Check sheet for the modelled part. Datum: model origin and axes. Units: mm. A direction names the side the tool comes from. Coordinates: 2 decimals unless noted, no trailing zeros. Loops run counter-clockwise (first coordinate to the right, second up) from the corner with the lowest first, then second, coordinate; pieces in that order, holes last. Notation, with made-up numbers: M -25,53 L -10,53 A26 ccw -10,92 Z; hole C -29,20 d11. An arc over 180 degrees is marked long. Write each question's results on one line, items separated by ' | '. Start each with the question number.
from build123d import *

# Parameters (mm, degrees)
BOSS_EXTRUDE1_DEPTH = 415.925
SKETCH2_R           = 3.429
CUT_EXTRUDE1_DEPTH  = 26.4


with BuildPart() as part:
    # Sketch1 → Boss-Extrude1 (new body)
    with BuildSketch(Plane.XY):
        with BuildLine():
            Line((-12.446, -12.7), (12.446, -12.7))
            ThreePointArc((12.446, -12.7), (12.625605122, -12.625605122), (12.7, -12.446))
            Line((12.7, -12.446), (12.7, 12.446))
            ThreePointArc((12.7, 12.446), (12.625605122, 12.625605122), (12.446, 12.7))
            Line((12.446, 12.7), (-12.446, 12.7))
            ThreePointArc((-12.446, 12.7), (-12.625605122, 12.625605122), (-12.7, 12.446))
            Line((-12.7, 12.446), (-12.7, -12.446))
            ThreePointArc((-12.7, -12.446), (-12.625605122, -12.625605122), (-12.446, -12.7))
        make_face()
        with BuildLine():
            Line((-11.1125, -9.5885), (-11.1125, 9.5885))
            ThreePointArc((-11.1125, 9.5885), (-10.666130735, 10.666130735), (-9.5885, 11.1125))
            Line((-9.5885, 11.1125), (9.5885, 11.1125))
            ThreePointArc((9.5885, 11.1125), (10.666130735, 10.666130735), (11.1125, 9.5885))
            Line((11.1125, 9.5885), (11.1125, -9.5885))
            ThreePointArc((11.1125, -9.5885), (10.666130735, -10.666130735), (9.5885, -11.1125))
            Line((9.5885, -11.1125), (-9.5885, -11.1125))
            ThreePointArc((-9.5885, -11.1125), (-10.666130735, -10.666130735), (-11.1125, -9.5885))
        make_face(mode=Mode.SUBTRACT)
    extrude(amount=BOSS_EXTRUDE1_DEPTH)

    # Sketch2 → Cut-Extrude1 (cut, through all)
    with BuildSketch(Plane.ZY.offset(12.7)):
        with Locations((371.475, 0)):
            Circle(SKETCH2_R)
        with Locations((358.775, 0)):
            Circle(SKETCH2_R)
        with Locations((346.075, 0)):
            Circle(SKETCH2_R)
        with Locations((12.7, 0)):
            Circle(SKETCH2_R)
        with Locations((25.4, 0)):
            Circle(SKETCH2_R)
        Polygon((415.925, 12.7), (371.930909488, -12.7), (415.925, -12.7), align=None)
        Polygon((0, 5.78069553), (4.844949149, 12.7), (0, 12.7), align=None)
    extrude(amount=-CUT_EXTRUDE1_DEPTH, mode=Mode.SUBTRACT)


solid = part.part
Item 1: Section check D-D (y = 0). State how many separate pieces and enclosed holes the cut face has, plus the area to 3 significant figures.
Item 2: Depth check by flat-ended pin: P1, Ø9, axis at y = 0, z = 346.075, coming from the -X side. Enter the tip coordinate at first touch or a pass-through.
Item 3: Section check B-B (x = -0.75). Record the cut outline in (y, z) (1 decimal).
Item 4: Thickness scan on line 1 (Y direction, x = 8, z = 144); line 2 (Y direction, x = 8, z = 375). Record the ranges inside material, lowest first.
Item 5: Release check for a two-part mould opening along Y. For faces 3 (the face through (-12.7, 0, 205)), 4 (the face through (0, 12.7, 208)), 5 (the face through (11.112, 0, 202)), 6 (the face through (-11.35, 0.06, 394.03)) record: +Y half, -Y half, draft (parallel to the pull), parting line (faces both ways), or undercut.
Item 6: Tool access check on faces 1 (the face through (-11.112, 0, 202)), 2 (the face through (-11.917, -1.313, 361.943)). Record the directions out of +Z, -Z, +X, -X, +Y, -Y that give a thin tool (end or side, any length) a straight path to the whole face; none if there is none.
Item 7: Section check C-C (z = 89). Record the cut outline in (x, y), plus the area to 3 significant figures.
Item 8: Section check A-A (z = 25.4). Record the cut outline in (x, y).
Computed values:
1) separate pieces: 12 | enclosed holes: 0 | area: 1,140 mm²
2) P1: stops at x = -12.7
3) outline: M -12.7,0 L -11.1,0 L -11.1,374.7 L -12.7,371.9 Z; M 11.1,3.7 L 12.7,4.8 L 12.7,415.9 L 11.1,413.2 Z
4) line 1: y = -12.7 to -11.11, 11.11 to 12.7 | line 2: y = 11.11 to 12.7
5) face 3: draft | face 4: +Y half | face 5: undercut | face 6: -Y half
6) face 1: +Z, -Z | face 2: +X, -X
7) outline: M -12.7,-12.45 A0.25 ccw -12.45,-12.7 L 12.45,-12.7 A0.25 ccw 12.7,-12.45 L 12.7,12.45 A0.25 ccw 12.45,12.7 L -12.45,12.7 A0.25 ccw -12.7,12.45 Z; hole M -11.11,-9.59 A1.52 ccw -9.59,-11.11 L 9.59,-11.11 A1.52 ccw 11.11,-9.59 L 11.11,9.59 A1.52 ccw 9.59,11.11 L -9.59,11.11 A1.52 ccw -11.11,9.59 Z | area: 153 mm²
8) outline: M -12.7,-12.45 A0.25 ccw -12.45,-12.7 L 12.45,-12.7 A0.25 ccw 12.7,-12.45 L 12.7,-3.43 L 11.11,-3.43 L 11.11,-9.59 A1.52 cw 9.59,-11.11 L -9.59,-11.11 A1.52 cw -11.11,-9.59 L -11.11,-3.43 L -12.7,-3.43 Z; M -12.7,3.43 L -11.11,3.43 L -11.11,9.59 A1.52 cw -9.59,11.11 L 9.59,11.11 A1.52 cw 11.11,9.59 L 11.11,3.43 L 12.7,3.43 L 12.7,12.45 A0.25 ccw 12.45,12.7 L -12.45,12.7 A0.25 ccw -12.7,12.45 Z
